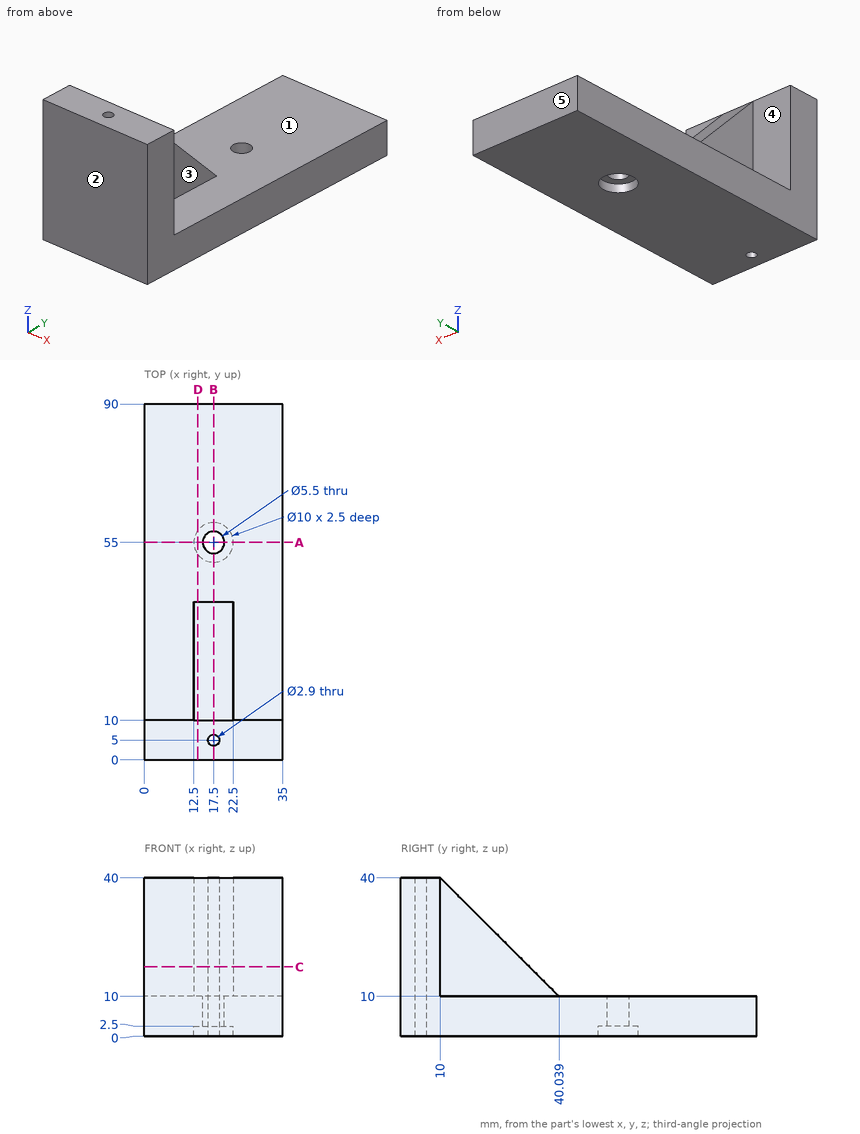
Verification items for this drawing (mm, ordinates from the low corner). A direction names the side the tool comes from. Coordinates: 2 decimals unless noted, no trailing zeros. Loops run counter-clockwise (first coordinate to the right, second up) from the corner with the lowest first, then second, coordinate; pieces in that order, holes last. Notation, with made-up numbers: (49.25, 52.5) - (84.25, 52.5) arc R21 cw to (84.25, 74.5) - close; hole circle Ø2 at (-25, 87). An arc over 180 degrees is marked (long way). Use one line per item in the form item = value. Start each with the question number.
Item 1: Gauge pin test, flat ends, axial feed: pin 1 (5 mm diameter, centred on x = 31, y = 46, fed in from +Z); pin 2 (1 mm diameter, centred on x = 5, z = 16.5, fed in from +Y); pin 3 (4 mm diameter, centred on x = 13, y = 20.5, fed in from -Z); pin 4 (4.5 mm diameter, centred on x = 17.5, y = 55, fed in from +Z). Record the tip position at first contact, or that the pin passes through.
Item 2: Section check B-B, the plane x = 17.5. Enter the section's corners in (y, z), and give its area (3 significant figures).
Item 3: Section check A-A, the plane y = 55. Enter the section's corners in (x, z), and give its area (3 significant figures).
Item 4: Section check D-D, the plane x = 13.5. Enter the section's corners in (y, z).
Item 5: Section check C-C, the plane z = 17.5. Enter the section's corners in (x, y), and give its area (3 significant figures).
Item 6: Tool access check on the marked faces 1, 2, 3, 4 and 5. Record the directions out of +Z, -Z, +X, -X, +Y, -Y that give a thin tool (end or side, any length) a straight path to the whole face; none if there is none.
Item 7: Thickness scan on probe 1 along Y at (x, z) = (17.5, 7); probe 2 along X at (y, z) = (55, 1.9); probe 3 along X at (y, z) = (5, 21.5). Record the ranges inside material, lowest first.
Computed:
q1.pin_1 = 10
q1.pin_2 = 10
q1.pin_3 = 0
q1.pin_4 = through
q2.outline = (0, 0) - (3.55, 0) - (3.55, 40) - (0, 40) - close; (6.45, 0) - (50, 0) - (50, 2.5) - (52.25, 2.5) - (52.25, 10) - (40.04, 10) - (10, 40) - (6.45, 40) - close; (57.75, 2.5) - (60, 2.5) - (60, 0) - (90, 0) - (90, 10) - (57.75, 10) - close
q2.area = 1,470 mm2
q3.outline = (0, 0) - (12.5, 0) - (12.5, 2.5) - (14.75, 2.5) - (14.75, 10) - (0, 10) - close; (20.25, 2.5) - (22.5, 2.5) - (22.5, 0) - (35, 0) - (35, 10) - (20.25, 10) - close
q3.area = 284 mm2
q4.outline = (0, 0) - (52, 0) - (52, 2.5) - (58, 2.5) - (58, 0) - (90, 0) - (90, 10) - (40.04, 10) - (10, 40) - (0, 40) - close
q5.outline = (0, 0) - (35, 0) - (35, 10) - (22.5, 10) - (22.5, 32.53) - (12.5, 32.53) - (12.5, 10) - (0, 10) - close; hole circle Ø2.9 at (17.5, 5)
q5.area = 569 mm2
q6.face_1 = +Z, +Y
q6.face_2 = +Z, -Z, +X, -X, -Y
q6.face_3 = +Z, +X, +Y
q6.face_4 = +Z, -X, +Y
q6.face_5 = +Z, -Z, +X, -X, +Y
q7.probe_1 = 0 to 3.55, 6.45 to 52.25, 57.75 to 90
q7.probe_2 = 0 to 12.5, 22.5 to 35
q7.probe_3 = 0 to 16.05, 18.95 to 35
